Could you check a few things on this drawing? It's one solid part, dimensions in mm from its lowest x, y, z. Coordinates: 2 decimals unless noted, no trailing zeros. Loops run counter-clockwise (first coordinate to the right, second up) from the corner with the lowest first, then second, coordinate; pieces in that order, holes last.
1) If I drill on line 1 along Y through (x, z) = (69, 0.7); line 2 along X through (y, z) = (77, 5); line 3 along X through (y, z) = (15, 3.1), over which ranges is the centre line in solid material (lowest first)?
2) Imagine slicing it at A-A on x = 17. Please give me the cut outline in (y, z).
3) Imagine slicing it at C-C on y = 83. Please give me the cut outline in (x, z), plus the area to 3 significant figures.
4) Will these pins go through, and if not, where does the flat tip stop? P1, Ø1.8, axis at x = 84, z = 4, coming from the +Y side; P2, Ø1.8, axis at x = 44, z = 2, coming from the -Y side; P3, Ø1.8, axis at y = 81, z = 4, coming from the -X side.
5) Imagine slicing it at B-B on z = 4.05. Please give me the cut outline in (x, y), plus the area to 3 significant figures.
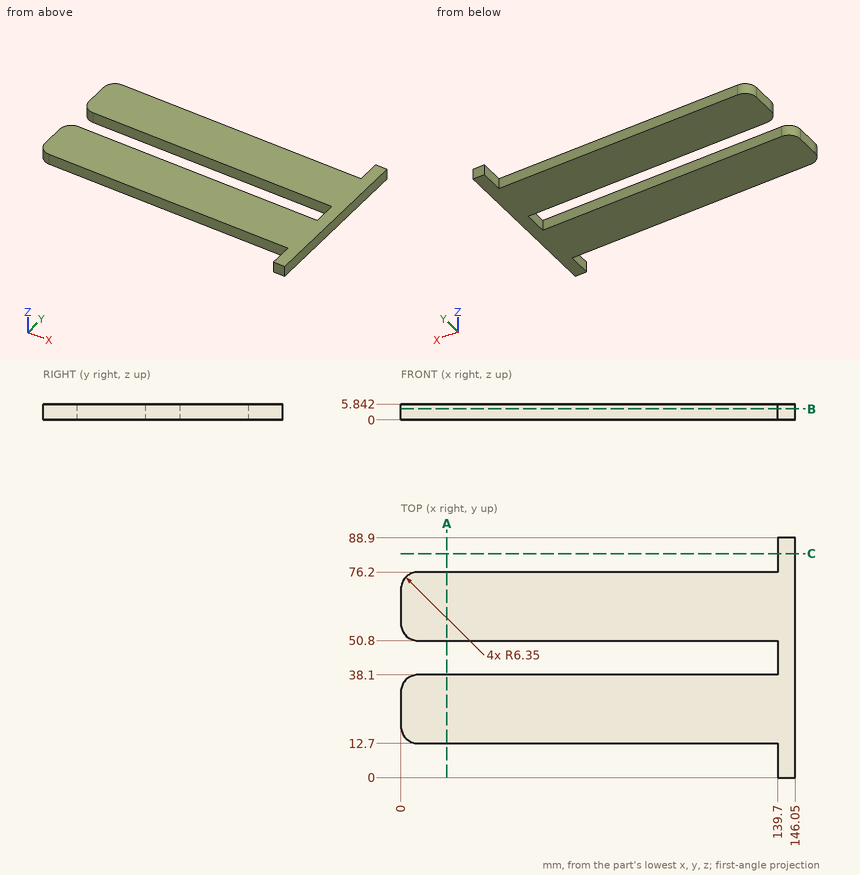
Filled in:
1. line 1: y = 12.7 to 38.1, 50.8 to 76.2
1. line 2: x = 139.7 to 146.05
1. line 3: x = 1.46 to 146.05
2. outline: (12.7, 0) - (38.1, 0) - (38.1, 5.84) - (12.7, 5.84) - close; (50.8, 0) - (76.2, 0) - (76.2, 5.84) - (50.8, 5.84) - close
3. outline: (139.7, 0) - (146.05, 0) - (146.05, 5.84) - (139.7, 5.84) - close
3. area: 37.1 mm2
4. P1: stops at y = 76.2
4. P2: stops at y = 12.7
4. P3: stops at x = 139.7
5. outline: (0, 19.05) arc R6.35 ccw to (6.35, 12.7) - (139.7, 12.7) - (139.7, 0) - (146.05, 0) - (146.05, 88.9) - (139.7, 88.9) - (139.7, 76.2) - (6.35, 76.2) arc R6.35 ccw to (0, 69.85) - (0, 57.15) arc R6.35 ccw to (6.35, 50.8) - (139.7, 50.8) - (139.7, 38.1) - (6.35, 38.1) arc R6.35 ccw to (0, 31.75) - close
5. area: 7,630 mm2
